Geometry: final body of the model. Coordinates: model frame, mm. Give positions to 0.01 mm unless a question says otherwise; leave off trailing zeros. Write each loop counter-clockwise with the first axis right and the second up, starting at its lowest first coordinate (ties: lowest second). Pieces come first, ordered by that corner, then holes.
```python
from build123d import *

# Parameters (mm, degrees)
SKETCH_1_R      = 2
EXTRUDE_1_DEPTH = 6


with BuildPart() as part:
    # Эскиз1 → Бобышка-Вытянуть1 (new body)
    with BuildSketch(Plane.XY):
        with BuildLine():
            Line((45, -21), (-45, -21))
            ThreePointArc((-45, -21), (-48.535533906, -19.535533906), (-50, -16))
            Line((-50, -16), (-50, 16))
            ThreePointArc((-50, 16), (-48.535533906, 19.535533906), (-45, 21))
            Line((-45, 21), (45, 21))
            ThreePointArc((45, 21), (48.535533906, 19.535533906), (50, 16))
            Line((50, 16), (50, -16))
            ThreePointArc((50, -16), (48.535533906, -19.535533906), (45, -21))
        make_face()
        with Locations((-40, 11)):
            Circle(SKETCH_1_R, mode=Mode.SUBTRACT)
        with Locations((-20, 11)):
            Circle(SKETCH_1_R, mode=Mode.SUBTRACT)
        with Locations(Location((-40, -11, 0), (0, 0, 180))):
            Circle(SKETCH_1_R, mode=Mode.SUBTRACT)
        with Locations(Location((-20, -11, 0), (0, 0, 180))):
            Circle(SKETCH_1_R, mode=Mode.SUBTRACT)
        with Locations((20, -11)):
            Circle(SKETCH_1_R, mode=Mode.SUBTRACT)
        with Locations((40, -11)):
            Circle(SKETCH_1_R, mode=Mode.SUBTRACT)
        with Locations(Location((40, 11, 0), (0, 0, 180))):
            Circle(SKETCH_1_R, mode=Mode.SUBTRACT)
        with Locations(Location((20, 11, 0), (0, 0, 180))):
            Circle(SKETCH_1_R, mode=Mode.SUBTRACT)
    extrude(amount=EXTRUDE_1_DEPTH)


solid = part.part
```
Item 1: Section C-C, the plane x = 40. Return the cut outline in (y, z), plus the area to 3 significant figures.
Found:
outline: (-21, 0) - (-13, 0) - (-13, 6) - (-21, 6) - close; (-9, 0) - (9, 0) - (9, 6) - (-9, 6) - close; (13, 0) - (21, 0) - (21, 6) - (13, 6) - close
area: 204 mm2
Item 2: Section A-A, the plane y = -11. Return the cut outline in (x, z), plus the area to 3 significant figures.
Found:
outline: (-50, 0) - (-42, 0) - (-42, 6) - (-50, 6) - close; (-38, 0) - (-22, 0) - (-22, 6) - (-38, 6) - close; (-18, 0) - (18, 0) - (18, 6) - (-18, 6) - close; (22, 0) - (38, 0) - (38, 6) - (22, 6) - close; (42, 0) - (50, 0) - (50, 6) - (42, 6) - close
area: 504 mm2
Item 3: Line query: L1, parallel to Y at x = -40, z = 5.1; L2, parallel to X at y = 12, z = 4.35; L3, parallel to X at y = 11.5, z = 1.5. Output: solid intervals per line, ascending.
Found:
L1: y = -21 to -13, -9 to 9, 13 to 21
L2: x = -50 to -41.73, -38.27 to -21.73, -18.27 to 18.27, 21.73 to 38.27, 41.73 to 50
L3: x = -50 to -41.94, -38.06 to -21.94, -18.06 to 18.06, 21.94 to 38.06, 41.94 to 50
Item 4: Pin query (flat end, axial travel): pin 1 Ø3 at (x, y) = (-20, -11) entering from +Z; pin 2 Ø4.5 at (x, y) = (20, -11) entering from -Z. Return the tip coordinate at first contact, or that it passes through.
Found:
pin 1: passes through
pin 2: stops at z = 0
Item 5: Pull-direction query (Y, two-part tool) for faces 1 (the face through (49, -19, 3)), 2 (the face through (-50, 0, 3)), 3 (the face through (21.474, 9.648, 2.958)); classes: +Y half, -Y half, draft (parallel to the pull), parting line (faces both ways), or undercut.
Found:
face 1: -Y half
face 2: draft
face 3: undercut
Item 6: Section B-B, the plane z = 1.6. State how many separate pieces and enclosed holes the cut face has, plus the area to 3 significant figures.
Found:
separate pieces: 1
enclosed holes: 8
area: 4,080 mm2
